Part model, mm, in its own coordinate system. Face numbers are marked on the shaded views. A direction names the side the tool comes from. Give positions to 0.01 mm unless a question says otherwise; leave off trailing zeros. Order: outer loops, then holes, each group sorted by start corner. A loop starts at its lowest first (then second) coordinate and runs counter-clockwise, first axis right, second up. Notation, with made-up numbers: (-13, 76) -> (30, 76) arc R22 ccw to (30, 101) -> close; hole circle Ø1 at (52, 50.5). An arc over 180 degrees is marked (long way). Write item = value, one per line. Start each with the question number.
Item 1: Pull direction X, two halves, no side cores. Call the marked faces 1 and 2: +X half, -X half, draft (parallel to the pull), parting line (faces both ways), or undercut.
Item 2: Flat gauge pins, fed straight in: P1, Ø0.9, axis at x = -5.5, z = 1, coming from the +Y side; P2, Ø1.5, axis at x = -1, z = 2.5, coming from the +Y side; P3, Ø0.9, axis at y = 7.5, z = 1.5, coming from the -X side. Where does each tip first touch, or does it go through?
Item 3: Tool access for the marked faces 3 and 4: list every direction of +Z, -Z, +X, -X, +Y, -Y with a clear straight run to the whole face (end or side of a thin tool).
Item 4: Band-saw the part on B-B on y = 42. Write the cut outline in (x, z), plus the area to 3 significant figures.
Item 5: Band-saw the part on A-A on x = 3.5. Write the cut outline in (y, z), plus the area to 3 significant figures.
Item 6: Drill centre lines: line 1 along X through (y, z) = (38, 1.15); line 2 along Y through (x, z) = (-2.5, 1.1); line 3 along Y through (x, z) = (-11.5, 1.5). Where is each one in solid material? Low to high.
Item 7: Band-saw the part on C-C on z = 1.05. Write the cut outline in (x, y), plus the area to 3 significant figures.
```python
from build123d import *

# Parameters (mm, degrees)
EXTRUDE_1_DEPTH = 3


with BuildPart() as part:
    # 草图2 → 凸台-拉伸1 (new body)
    with BuildSketch(Plane.XY):
        with BuildLine():
            Line((2.047890023, 48.855305477), (8, 48.855305477))
            Line((8, 48.855305477), (8, 51.855305477))
            Line((8, 51.855305477), (16, 51.855305477))
            Line((16, 51.855305477), (16, 8.855305477))
            Line((16, 8.855305477), (8, 8.855305477))
            Line((8, 8.855305477), (8, 5.855305477))
            Line((8, 5.855305477), (0.390512484, 5.855305477))
            ThreePointArc((0.390512484, 5.855305477), (0, 8.905305477), (-0.390512484, 5.855305477))
            Line((-0.390512484, 5.855305477), (-8, 5.855305477))
            Line((-8, 5.855305477), (-8, 8.855305477))
            Line((-8, 8.855305477), (-16, 8.855305477))
            Line((-16, 8.855305477), (-16, 51.855305477))
            Line((-16, 51.855305477), (-8, 51.855305477))
            Line((-8, 51.855305477), (-8, 48.855305477))
            Line((-8, 48.855305477), (-2.047890023, 48.855305477))
            Line((-2.047890023, 48.855305477), (-2.047890023, 43.855305477))
            Line((-2.047890023, 43.855305477), (-4, 43.855305477))
            Line((-4, 43.855305477), (-4, 40.855305477))
            Line((-4, 40.855305477), (-2, 40.855305477))
            Line((-2, 40.855305477), (-2, 36.855305477))
            Line((-2, 36.855305477), (2, 36.855305477))
            Line((2, 36.855305477), (2, 40.855305477))
            Line((2, 40.855305477), (4, 40.855305477))
            Line((4, 40.855305477), (4, 43.855305477))
            Line((4, 43.855305477), (2.047890023, 43.855305477))
            Line((2.047890023, 43.855305477), (2.047890023, 48.855305477))
        make_face()
    extrude(amount=EXTRUDE_1_DEPTH)


solid = part.part
```
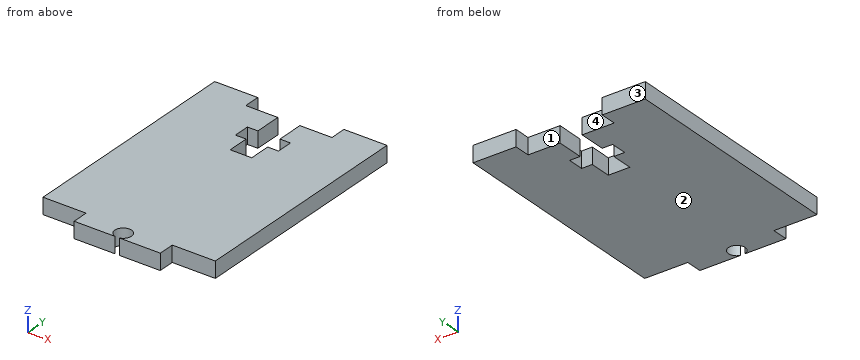
Values found:
q1.face_1 = undercut
q1.face_2 = draft
q2.P1 = 48.86
q2.P2 = 36.86
q2.P3 = -8
q3.face_3 = +Z, -Z, +X, -X, +Y
q3.face_4 = +Z, -Z, +Y
q4.outline = (-16, 0) -> (-4, 0) -> (-4, 3) -> (-16, 3) -> close; (4, 0) -> (16, 0) -> (16, 3) -> (4, 3) -> close
q4.area = 72.0 mm^2
q5.outline = (5.86, 0) -> (40.86, 0) -> (40.86, 3) -> (5.86, 3) -> close; (43.86, 0) -> (48.86, 0) -> (48.86, 3) -> (43.86, 3) -> close
q5.area = 120 mm^2
q6.line_1 = -16 to -2, 2 to 16
q6.line_2 = 5.86 to 40.86, 43.86 to 48.86
q6.line_3 = 8.86 to 51.86
q7.outline = (-16, 8.86) -> (-8, 8.86) -> (-8, 5.86) -> (-0.39, 5.86) arc R1.55 cw (long way) to (0.39, 5.86) -> (8, 5.86) -> (8, 8.86) -> (16, 8.86) -> (16, 51.86) -> (8, 51.86) -> (8, 48.86) -> (2.05, 48.86) -> (2.05, 43.86) -> (4, 43.86) -> (4, 40.86) -> (2, 40.86) -> (2, 36.86) -> (-2, 36.86) -> (-2, 40.86) -> (-4, 40.86) -> (-4, 43.86) -> (-2.05, 43.86) -> (-2.05, 48.86) -> (-8, 48.86) -> (-8, 51.86) -> (-16, 51.86) -> close
q7.area = 1,310 mm^2
